Here's how the part is built. I have some questions about the finished solid (model axes, mm). Give positions to 0.01 mm unless a question says otherwise; leave off trailing zeros. Loops run counter-clockwise (first coordinate to the right, second up) from the corner with the lowest first, then second, coordinate; pieces in that order, holes last.
Q1. I need wall thicknesses on probe 1 along X at (y, z) = (-358, 5.1); probe 2 along Y at (x, z) = (-84, 1.3). Which ranges of each line are inside material? Lowest first, please.
Q2. Suppose I cut it at B-B (z = 1.05). List the corners of the cut face in (x, y) for me, and give its area (3 significant figures).
Q3. Suppose I cut it at A-A (y = -436). List the corners of the cut face in (x, z) for me.
Q4. Suppose I cut it at C-C (x = -38). List the corners of the cut face in (y, z) for me.
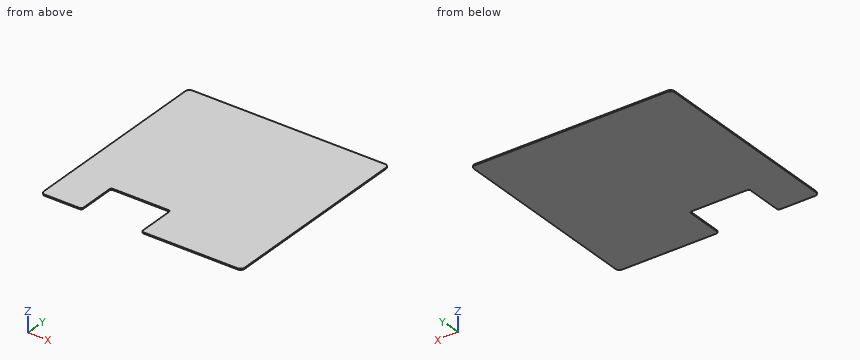
```python
from build123d import *

# Parameters (mm, degrees)
SKETCH1_W           = 1010
SKETCH1_H           = 1010
BOSS_EXTRUDE1_DEPTH = 6
SKETCH2_W           = 300
SKETCH2_H           = 200
CUT_EXTRUDE1_DEPTH  = 6
FILLET2_R           = 20
FILLET3_R           = 10


with BuildPart() as part:
    # Sketch1 → Boss-Extrude1 (new body)
    with BuildSketch(Plane.XY):
        Rectangle(SKETCH1_W, SKETCH1_H)
    extrude(amount=BOSS_EXTRUDE1_DEPTH)

    # Sketch2 → Cut-Extrude1 (cut)
    with BuildSketch(Plane.XY.offset(6)):
        with Locations((-150, -405)):
            Rectangle(SKETCH2_W, SKETCH2_H)
    extrude(amount=-CUT_EXTRUDE1_DEPTH, mode=Mode.SUBTRACT)

    # Fillet2
    fillet2_edges = [part.edges().sort_by_distance(p)[0] for p in [
        (-505, 505, 3),
        (505, 505, 3),
        (505, -505, 3),
        (-505, -505, 3),
    ]]
    fillet(fillet2_edges, radius=FILLET2_R)

    # Fillet3
    fillet3_edges = [part.edges().sort_by_distance(p)[0] for p in [
        (-300, -505, 3),
        (-300, -305, 3),
        (0, -305, 3),
        (0, -505, 3),
    ]]
    fillet(fillet3_edges, radius=FILLET3_R)


solid = part.part
```
Solutions:
1. probe 1: x = -505 to -300, 0 to 505
1. probe 2: y = -305 to 505
2. outline: (-505, -485) arc R20 ccw to (-485, -505) - (-310, -505) arc R10 ccw to (-300, -495) - (-300, -315) arc R10 cw to (-290, -305) - (-10, -305) arc R10 cw to (0, -315) - (0, -495) arc R10 ccw to (10, -505) - (485, -505) arc R20 ccw to (505, -485) - (505, 485) arc R20 ccw to (485, 505) - (-485, 505) arc R20 ccw to (-505, 485) - close
2. area: 960,000 mm2
3. outline: (-505, 0) - (-300, 0) - (-300, 6) - (-505, 6) - close; (0, 0) - (505, 0) - (505, 6) - (0, 6) - close
4. outline: (-305, 0) - (505, 0) - (505, 6) - (-305, 6) - close
